Build history of the part. All positions in model axes, mm. Face numbers are marked on the shaded views. A direction names the side the tool comes from. Give positions to 0.01 mm unless a question says otherwise; leave off trailing zeros. Write each loop counter-clockwise with the first axis right and the second up, starting at its lowest first coordinate (ties: lowest second). Pieces come first, ordered by that corner, then holes. Notation, with made-up numbers: (-19, 55.25) -> (24, 55.25) arc R18 cw to (24, 81.25) -> close; hole circle Ø2 at (18.25, -15.75). An arc over 180 degrees is marked (long way). Write item = value, one per line. Start each with the question number.
Q1. Saw through at A-A, the plane x = 17.5. List the corners of the cut face in (y, z) (3 decimals).
Q2. Wall check: line 1 (X direction, y = -13, z = -7.75); line 2 (X direction, y = 6.5, z = -6.5); line 3 (Z direction, x = -17.5, y = 15.75). Give the ranges that are in metal, low to high.
Q3. Mould opens along Y. For the marked faces 1, 2 and 3 say: pulls with the +Y half, pulls with the -Y half, needs draft (parallel to the pull), parting line crosses it, or undercut.
Q4. Tool access for the marked faces 4 and 5: list every direction of +Z, -Z, +X, -X, +Y, -Y with a clear straight run to the whole face (end or side of a thin tool).
Q5. Saw through at D-D, the plane x = 0. List the corners of the cut face in (y, z).
Q6. Saw through at C-C, the plane y = 4. List the corners of the cut face in (x, z).
Q7. Drop flat-ended pins along their axis: P1, Ø6, axis at x = 17.5, z = -8, coming from the +Y side; P2, Ø11, axis at x = -3.5, y = 4.5, coming from the +Z side; P3, Ø6, axis at x = 17.5, z = -9.5, coming from the +Y side. Give the stop position or say it passes through.
Q8. Saw through at B-B, the plane z = -8. List the corners of the cut face in (x, y) (3 decimals).
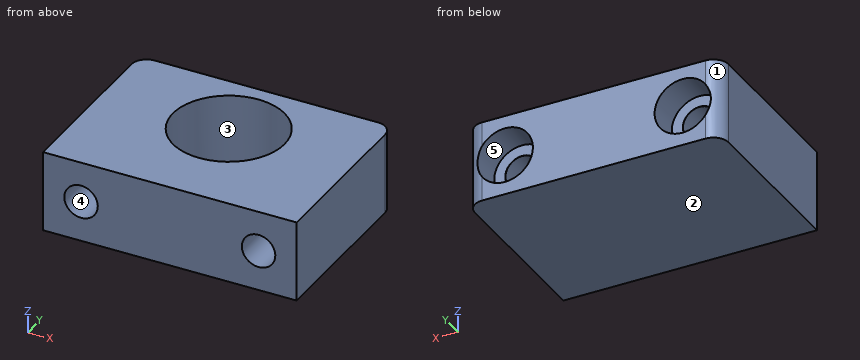
from build123d import *

# Parameters (mm, degrees)
EXTRUDE_349_DEPTH        = 16
HOLE_WIZARD_6_AT_2_COUNT = 2
HOLE_WIZARD_6_AT_2_PITCH = 35
SKETCH_14_R              = 11
CUT_EXTRUDE_608_DEPTH    = 14


with BuildPart() as part:
    # Эскиз8 → Extrude 349 (new body)
    with BuildSketch(Plane.XY):
        with BuildLine():
            Line((-22, 18), (22, 18))
            ThreePointArc((22, 18), (24.121320344, 17.121320344), (25, 15))
            Line((25, 15), (25, -18))
            Line((25, -18), (-25, -18))
            Line((-25, -18), (-25, 15))
            ThreePointArc((-25, 15), (-24.121320344, 17.121320344), (-22, 18))
        make_face()
    extrude(amount=-EXTRUDE_349_DEPTH)

    # Эскиз11 → Крепление-М6 (revolve, cut)
    with BuildSketch(Plane(origin=(-17.5, 18, -8), x_dir=(0, 0, 1), z_dir=(1, 0, 0))):
        Polygon((0, 0), (0, 36), (3.3, 36), (3.3, 6.425), (3.325, 6.4), (5.5, 6.4), (5.5, 0), align=None)
    hole_wizard_6 = revolve(axis=Axis((-17.5, 24.35, -8), (0, -1, 0)), mode=Mode.SUBTRACT)

    # Крепление-М6 at 2: Крепление-М6 ×2
    with Locations(*[(i * HOLE_WIZARD_6_AT_2_PITCH, 0, 0) for i in range(1, HOLE_WIZARD_6_AT_2_COUNT)]):
        add(hole_wizard_6, mode=Mode.SUBTRACT)

    # Эскиз14 → Вырез-608 (cut)
    with BuildSketch(Plane.XY):
        with Locations((0, 4)):
            Circle(SKETCH_14_R)
    extrude(amount=-CUT_EXTRUDE_608_DEPTH, mode=Mode.SUBTRACT)


solid = part.part
Report:
q1.outline = (-18, -16) -> (18, -16) -> (18, -13.5) -> (11.6, -13.5) -> (11.6, -11.325) -> (11.575, -11.3) -> (-18, -11.3) -> close; (-18, -4.7) -> (11.575, -4.7) -> (11.6, -4.675) -> (11.6, -2.5) -> (18, -2.5) -> (18, 0) -> (-18, 0) -> close
q2.line_1 = -25 to -20.79, -14.21 to 14.21, 20.79 to 25
q2.line_2 = -25 to -20.44, -14.56 to -10.71, 10.71 to 14.56, 20.44 to 25
q2.line_3 = -16 to -13.5, -2.5 to 0
q3.face_1 = pulls with the +Y half
q3.face_2 = needs draft
q3.face_3 = undercut
q4.face_4 = +Y, -Y
q4.face_5 = +Y
q5.outline = (-18, -16) -> (18, -16) -> (18, 0) -> (15, 0) -> (15, -14) -> (-7, -14) -> (-7, 0) -> (-18, 0) -> close
q6.outline = (-25, -16) -> (25, -16) -> (25, 0) -> (11, 0) -> (11, -14) -> (-11, -14) -> (-11, 0) -> (-25, 0) -> close; hole circle Ø6.6 at (-17.5, -8); hole circle Ø6.6 at (17.5, -8)
q7.P1 = through
q7.P2 = -14
q7.P3 = 11.6
q8.outline = (-25, -18) -> (-20.8, -18) -> (-20.8, 11.575) -> (-20.825, 11.6) -> (-23, 11.6) -> (-23, 17.828) arc R3 ccw to (-25, 15) -> close; (-14.2, -18) -> (14.2, -18) -> (14.2, 11.575) -> (14.175, 11.6) -> (12, 11.6) -> (12, 18) -> (-12, 18) -> (-12, 11.6) -> (-14.175, 11.6) -> (-14.2, 11.575) -> close; (20.8, -18) -> (25, -18) -> (25, 15) arc R3 ccw to (23, 17.828) -> (23, 11.6) -> (20.825, 11.6) -> (20.8, 11.575) -> close; hole circle Ø22 at (0, 4)
